Read the model definition and answer for the solid it produces. Units are mm, in the model's axes. Give positions to 0.01 mm unless a question says otherwise; leave off trailing zeros. Order: outer loops, then holes, each group sorted by start corner. A loop starts at its lowest first (then second) coordinate and runs counter-clockwise, first axis right, second up. Notation, with made-up numbers: M 73,20 L 113,20 A29 ccw 113,50 Z; hole C 15,57 d11. An arc over 180 degrees is marked long. One line per item, written item: value.
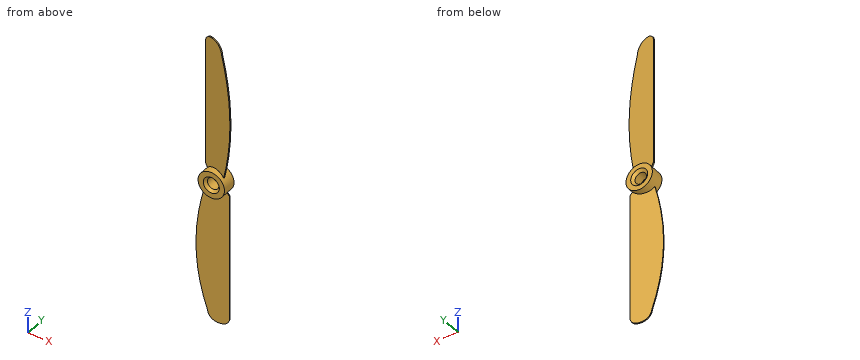
from build123d import *
from OCP.BRepFilletAPI import BRepFilletAPI_MakeChamfer

# Parameters (mm, degrees)
SKETCH_1_R               = 5.75
EXTRUDE_1_DEPTH          = 3
EXTRUDE_2_DEPTH          = 0.25
PATTERN_CIRCULAR_1_COUNT = 2
SKETCH_4_R               = 2.5
CUT_EXTRUDE_1_DEPTH      = 65.222479954
CHAMFER_1_SIZE           = 1
CHAMFER_1_SIZE2          = 1.191753593


with BuildPart() as part:
    # 草图1 → 凸台-拉伸1 (new, symmetric)
    with BuildSketch(Plane(origin=(0, 0, 0), x_dir=(1, 0, 0), z_dir=(0, 1, 0))):
        with Locations(Location((0, 0, 0), (0, 0, 270))):
            Circle(SKETCH_1_R)
    extrude(amount=EXTRUDE_1_DEPTH, both=True)

    # 草图3 → 凸台-拉伸2 (add, symmetric)
    with BuildSketch(Plane(origin=(0, 0, 0), x_dir=(0.9743700647852351, -0.22495105434386545, 0), z_dir=(-0.22495105434386545, -0.9743700647852351, 0))):
        with BuildLine():
            Line((-3.916367875, 3.295399757), (-5.31388764, 5.389585316))
            Line((-5.31388764, 5.389585316), (-5.31388764, 60.5))
            ThreePointArc((-5.31388764, 60.5), (-4.435207984, 62.621320344), (-2.31388764, 63.5))
            Line((-2.31388764, 63.5), (-1.829824276, 63.5))
            ThreePointArc((-1.829824276, 63.5), (1.545488809, 62.188802187), (3.15052064, 58.942904631))
            add(Edge.make_bspline(
                [(3.15052064, 58.942904631), (11.816057199, 30.493674225), (3.76071755, 1.848135525)],
                knots=[0, 0, 0, 1, 1, 1], degree=2))
            add(Edge.make_bspline(
                [(-3.916367875, 3.295399757), (0.478704758, 7.563280094), (3.76071755, 1.848135525)],
                knots=[0, 0, 0, 1, 1, 1], degree=2))
        make_face()
    extrude_2 = extrude(amount=EXTRUDE_2_DEPTH, both=True)

    # 阵列(圆周)1: 凸台-拉伸2 ×2 about axis
    pattern_circular_1_axis = Axis((0, -3, 0), (0, 1, 0))
    for i in range(1, PATTERN_CIRCULAR_1_COUNT):
        add(extrude_2.rotate(pattern_circular_1_axis, i * 360 / PATTERN_CIRCULAR_1_COUNT))

    # 草图4 → 切除-拉伸1 (cut, through all)
    with BuildSketch(Plane.XZ.offset(3)):
        with Locations(Location((0, 0, 0), (0, 0, 270))):
            Circle(SKETCH_4_R)
    extrude(amount=-CUT_EXTRUDE_1_DEPTH, mode=Mode.SUBTRACT)

    # 倒角1: one chamfer whose edges measure the first distance from different faces: ONE call of the kernel's chamfer builder (chamfer() names one face for all edges)
    chamfer_1_edges_1 = [part.edges().sort_by_distance(p)[0] for p in [
        (0, 3, 2.5),
    ]]
    chamfer_1_side_1 = [part.faces().sort_by_distance(p)[0] for p in [
        (0, 0, 2.5),
    ]]
    chamfer_1_edges_2 = [part.edges().sort_by_distance(p)[0] for p in [
        (0, -3, 2.5),
    ]]
    chamfer_1_side_2 = [part.faces().sort_by_distance(p)[0] for p in [
        (0, -3, -5.58736544),
    ]]
    chamfer_1 = BRepFilletAPI_MakeChamfer(part.part.solid().wrapped)
    for e in chamfer_1_edges_1:
        chamfer_1.Add(CHAMFER_1_SIZE, CHAMFER_1_SIZE2, e.wrapped, chamfer_1_side_1[0].wrapped)  # the first distance lies on this face
    for e in chamfer_1_edges_2:
        chamfer_1.Add(CHAMFER_1_SIZE, CHAMFER_1_SIZE2, e.wrapped, chamfer_1_side_2[0].wrapped)  # the first distance lies on this face
    add(Compound.cast(chamfer_1.Shape()), mode=Mode.REPLACE)


solid = part.part
1) Consider probe 1 along X at (y, z) = (0.8, 0); probe 2 along Z at (x, y) = (-1.75, 1); probe 3 along Z at (x, y) = (0, 2.25). Determine where each line is inside the solid, lowest interval first.
Reported:
probe 1: x = -5.75 to -2.5, 2.5 to 5.75
probe 2: z = -5.48 to -1.79, 1.79 to 5.48
probe 3: z = -5.75 to -2.8, 2.8 to 5.75
2) Find section A-A, the plane z = 0. Write down the section's boundary in (x, y).
Reported:
outline: M -5.75,-3 L -3.5,-3 L -2.5,-1.81 L -2.5,2 L -3.69,3 L -5.75,3 Z; M 2.5,-1.81 L 3.5,-3 L 5.75,-3 L 5.75,3 L 3.69,3 L 2.5,2 Z
3) Each of these flat-tipped pins is pushed along its axis until it touches: pin 1 Ø5 at (x, z) = (-1.5, 19) entering from -Y; pin 2 Ø4 at (x, z) = (0.5, 43) entering from -Y. Where does it stop, or does it pass through?
Reported:
pin 1: stops at y = -0.49
pin 2: stops at y = -0.83
